Input: part model. Units: mm. Frame: model coordinates. Face numbers are marked on the shaded views. Coordinates: 2 decimals unless noted, no trailing zeros. Loops run counter-clockwise (first coordinate to the right, second up) from the corner with the lowest first, then second, coordinate; pieces in that order, holes last. Notation, with made-up numbers: (74, -14.75) -> (109, -14.75) arc R9 cw to (109, -7.75) -> close; hole circle Ø8 at (41, 74.5). An arc over 180 degrees is marked (long way). Answer as a JSON object with one key per item and string values.
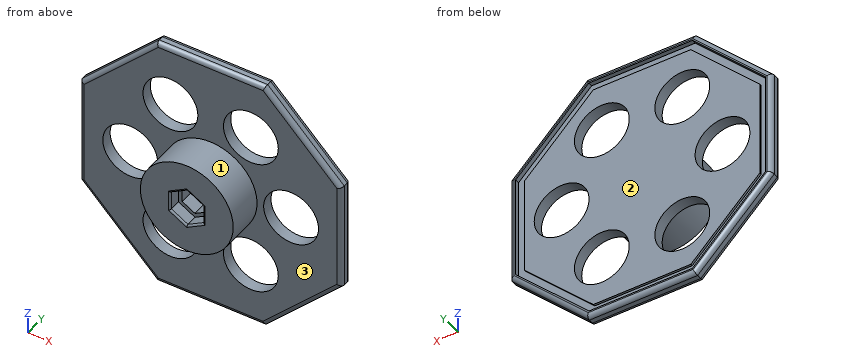
Autodesk Inventor part; units mm, degrees
ref_plane "YZ Plane" through (0, 0, 0) normal (1, 0, 0) x (0, 1, 0)
ref_plane "XZ Plane" through (0, 0, 0) normal (0, 1, 0) x (-1, 0, 0)
ref_plane "XY Plane" through (0, 0, 0) normal (0, 0, 1) x (1, 0, 0)
sketch "스케치3" plane through (0, 0, 0) normal (0, 1, 0) x (-1, 0, 0)
  line L0 (35.7919, -14.8255) -> (14.8255, -35.7919)
  line L1 (14.8255, -35.7919) -> (-14.8255, -35.7919)
  line L2 (-14.8255, -35.7919) -> (-35.7919, -14.8255)
  line L3 (-35.7919, -14.8255) -> (-35.7919, 14.8255)
  line L4 (-35.7919, 14.8255) -> (-14.8255, 35.7919)
  line L5 (-14.8255, 35.7919) -> (14.8255, 35.7919)
  line L6 (14.8255, 35.7919) -> (35.7919, 14.8255)
  line L7 (35.7919, 14.8255) -> (35.7919, -14.8255)
  line L8 (32.5919, -13.5) -> (13.5, -32.5919)
  line L9 (13.5, -32.5919) -> (-13.5, -32.5919)
  line L10 (-13.5, -32.5919) -> (-32.5919, -13.5)
  line L11 (-32.5919, -13.5) -> (-32.5919, 13.5)
  line L12 (-32.5919, 13.5) -> (-13.5, 32.5919)
  line L13 (-13.5, 32.5919) -> (13.5, 32.5919)
  line L14 (13.5, 32.5919) -> (32.5919, 13.5)
  line L15 (32.5919, 13.5) -> (32.5919, -13.5)
  point P0 (0, 0)
  point P1 (0, 0)
  point P2 (0, 0)
  point P3 (0, 0)
  dimension "d43" = 27
  dimension "d44" = 3.2
extrude "돌출2" add sketch "스케치3" along normal blind 3.7 contours L0 L1 L2 L3 L4 L5 L6 L7 | L8 L9 L10 L11 L12 L13 L14 L15
sketch "스케치4" plane through (0, 3.7, 0) normal (0, 1, 0) x (1, 0, 0)
  line L0 (13.5, -32.5919) -> (-13.5, -32.5919)
  line L1 (-13.5, -32.5919) -> (-32.5919, -13.5)
  line L2 (-32.5919, -13.5) -> (-32.5919, 13.5)
  line L3 (-32.5919, 13.5) -> (-13.5, 32.5919)
  line L4 (-13.5, 32.5919) -> (13.5, 32.5919)
  line L5 (13.5, 32.5919) -> (32.5919, 13.5)
  line L6 (32.5919, 13.5) -> (32.5919, -13.5)
  line L7 (32.5919, -13.5) -> (13.5, -32.5919)
  line L8 (-14.1627, 34.1919) -> (14.1627, 34.1919)
  line L9 (14.1627, 34.1919) -> (34.1919, 14.1627)
  line L10 (34.1919, 14.1627) -> (34.1919, -14.1627)
  line L11 (34.1919, -14.1627) -> (14.1627, -34.1919)
  line L12 (14.1627, -34.1919) -> (-14.1627, -34.1919)
  line L13 (-14.1627, -34.1919) -> (-34.1919, -14.1627)
  line L14 (-34.1919, -14.1627) -> (-34.1919, 14.1627)
  line L15 (-34.1919, 14.1627) -> (-14.1627, 34.1919)
  line L16 (-13.3343, 32.1919) -> (13.3343, 32.1919)
  line L17 (13.3343, 32.1919) -> (32.1919, 13.3343)
  line L18 (32.1919, 13.3343) -> (32.1919, -13.3343)
  line L19 (32.1919, -13.3343) -> (13.3343, -32.1919)
  line L20 (13.3343, -32.1919) -> (-13.3343, -32.1919)
  line L21 (-13.3343, -32.1919) -> (-32.1919, -13.3343)
  line L22 (-32.1919, -13.3343) -> (-32.1919, 13.3343)
  line L23 (-32.1919, 13.3343) -> (-13.3343, 32.1919)
  line L24 (-35.7919, 14.8255) -> (-35.7919, -14.8255)
  point P0 (0, 0)
  point P1 (0, 0)
  point P2 (0, 0)
  point P3 (0, 0)
  dimension "d7" = 27
  dimension "d60" = 1.6
  dimension "d61" = 2
extrude "돌출3" cut sketch "스케치4" against normal blind 1.2 contours L0 L1 L2 L3 L4 L5 L6 L7 | L8 L9 L10 L11 L12 L13 L14 L15 | L16 L17 L18 L19 L20 L21 L22 L23
sketch "스케치9" plane through (0, 2.5, 0) normal (0, 1, 0) x (1, 0, 0)
  line L0 (-13.3343, 32.1919) -> (13.3343, 32.1919)
  line L1 (13.3343, 32.1919) -> (32.1919, 13.3343)
  line L2 (32.1919, 13.3343) -> (32.1919, -13.3343)
  line L3 (32.1919, -13.3343) -> (13.3343, -32.1919)
  line L4 (13.3343, -32.1919) -> (-13.3343, -32.1919)
  line L5 (-13.3343, -32.1919) -> (-32.1919, -13.3343)
  line L6 (-32.1919, -13.3343) -> (-32.1919, 13.3343)
  line L7 (-32.1919, 13.3343) -> (-13.3343, 32.1919)
  line L8 (-14.1627, 34.1919) -> (14.1627, 34.1919)
  line L9 (-12.0917, 29.1919) -> (12.0917, 29.1919)
  line L10 (12.0917, 29.1919) -> (29.1919, 12.0917)
  line L11 (29.1919, 12.0917) -> (29.1919, -12.0917)
  line L12 (29.1919, -12.0917) -> (12.0917, -29.1919)
  line L13 (12.0917, -29.1919) -> (-12.0917, -29.1919)
  line L14 (-12.0917, -29.1919) -> (-29.1919, -12.0917)
  line L15 (-29.1919, -12.0917) -> (-29.1919, 12.0917)
  line L16 (-29.1919, 12.0917) -> (-12.0917, 29.1919)
  point P0 (0, 0)
  point P1 (0, 0)
  point P2 (0, 0)
  dimension "d46" = 2
  dimension "d47" = 3
extrude "돌출8" add sketch "스케치9" along normal blind 0.6 contours L0 L1 L2 L3 L4 L5 L6 L7 | L9 L10 L11 L12 L13 L14 L15 L16
fillet "모깎기1" radius 1.2 16 edges at (-35.7919, 3.7, 0) (-25.3087, 3.7, 25.3087) (0, 3.7, 35.7919) (25.3087, 3.7, 25.3087) (35.7919, 3.7, 0) (25.3087, 3.7, -25.3087) (0, 3.7, -35.7919) (-25.3087, 3.7, -25.3087) (25.3087, 0, 25.3087) (0, 0, 35.7919) (-25.3087, 0, 25.3087) (-35.7919, 0, 0) (-25.3087, 0, -25.3087) (0, 0, -35.7919) (25.3087, 0, -25.3087) (35.7919, 0, 0)
sketch "스케치11" plane through (0, 0, 0) normal (0, -1, 0) x (1, 0, 0)
  circle A0 centre (0, 0) radius 12.7
  dimension "d62" = 25.4
extrude "돌출11" add sketch "스케치11" along normal blind 10.16
sketch "스케치12" plane through (0, -10.16, 0) normal (0, -1, 0) x (1, 0, 0)
  circle A0 centre (0, 0) radius 4.5
  line L0 (4.5, 2.5981) -> (4.5, -2.5981)
  line L1 (4.5, -2.5981) -> (0, -5.1962)
  line L2 (0, -5.1962) -> (-4.5, -2.5981)
  line L3 (-4.5, -2.5981) -> (-4.5, 2.5981)
  line L4 (-4.5, 2.5981) -> (0, 5.1962)
  line L5 (0, 5.1962) -> (4.5, 2.5981)
  point P0 (2.25, 3.8971)
  point P1 (-2.25, 3.8971)
  point P2 (4.5, 0)
  point P3 (-4.5, 0)
  point P4 (-2.25, -3.8971)
  point P5 (2.25, -3.8971)
  dimension "d65" = 9
extrude "돌출12" cut sketch "스케치12" against normal blind 12
sketch "스케치13" plane through (0, 0, 0) normal (0, -1, 0) x (1, 0, 0)
  circle A0 centre (-22, 0) radius 7.5
  circle A1 centre (-11, -19.0526) radius 7.5
  circle A2 centre (11, -19.0526) radius 7.5
  circle A3 centre (22, 0) radius 7.5
  circle A4 centre (11, 19.0526) radius 7.5
  circle A5 centre (-11, 19.0526) radius 7.5
  point P0 (0, 0)
  dimension "d70" = 15
  dimension "d71" = 22
  dimension "d74" = 360
extrude "돌출13" cut sketch "스케치13" against normal up to surface (3.1 mm away)
sketch "스케치18" plane through (0, 1.84, 0) normal (0, -1, 0) x (1, 0, 0)
  line L0 (4.5, 2.5981) -> (4.5, -2.5981)
  line L1 (0, 5.1962) -> (4.5, 2.5981)
  line L2 (-4.5, 2.5981) -> (0, 5.1962)
  line L3 (-4.5, -2.5981) -> (-4.5, 2.5981)
  line L4 (0, -5.1962) -> (-4.5, -2.5981)
  line L5 (4.5, -2.5981) -> (0, -5.1962)
  line L6 (3.5, 2.0207) -> (3.5, -2.0207)
  line L7 (3.5, -2.0207) -> (0, -4.0415)
  line L8 (0, -4.0415) -> (-3.5, -2.0207)
  line L9 (-3.5, -2.0207) -> (-3.5, 2.0207)
  line L10 (-3.5, 2.0207) -> (0, 4.0415)
  line L11 (0, 4.0415) -> (3.5, 2.0207)
  point P0 (0, 0)
  point P1 (0, 0)
  dimension "d116" = 1
extrude "돌출14" add sketch "스케치18" along normal blind 8.5
fillet "모깎기2" radius 0.5 6 edges at (2.25, -10.16, 3.8971) (-2.25, -10.16, 3.8971) (4.5, -10.16, 0) (2.25, -10.16, -3.8971) (-2.25, -10.16, -3.8971) (-4.5, -10.16, 0)
equation "\"d85\" = 55deg"
equation "\"d105\" = 55deg"
properties part number "OV-PAM_top_2"
1. Section query B-B (x = -11). Return loops of the section in (y, z), plus the area to 3 significant figures.
Reply:
{"outline": "(-10.16, -6.35) -> (0, -6.35) -> (0, -11.55) -> (3.1, -11.55) -> (3.1, 11.55) -> (0, 11.55) -> (0, 6.35) -> (-10.16, 6.35) -> close; (0, -34.59) arc R1.2 ccw to (1.2, -35.79) -> (2.5, -35.79) arc R1.2 ccw to (3.7, -34.59) -> (3.7, -34.19) -> (2.5, -34.19) -> (2.5, -32.19) -> (3.1, -32.19) -> (3.1, -26.55) -> (0, -26.55) -> close; (0, 26.55) -> (3.1, 26.55) -> (3.1, 32.19) -> (2.5, 32.19) -> (2.5, 34.19) -> (3.7, 34.19) -> (3.7, 34.59) arc R1.2 ccw to (2.5, 35.79) -> (1.2, 35.79) arc R1.2 ccw to (0, 34.59) -> close", "area": "256 mm2"}
2. Section query C-C (z = 10). Return loops of the section in (x, y).
Reply:
{"outline": "(-35.79, 1.2) arc R1.2 ccw to (-34.59, 0) -> (-7.83, 0) -> (-7.83, -10.16) -> (7.83, -10.16) -> (7.83, 0) -> (34.59, 0) arc R1.2 ccw to (35.79, 1.2) -> (35.79, 2.5) arc R1.2 ccw to (34.59, 3.7) -> (34.19, 3.7) -> (34.19, 2.5) -> (32.19, 2.5) -> (32.19, 3.1) -> (-32.19, 3.1) -> (-32.19, 2.5) -> (-34.19, 2.5) -> (-34.19, 3.7) -> (-34.59, 3.7) arc R1.2 ccw to (-35.79, 2.5) -> close"}
3. Line query: line 1 along Z through (x, y) = (11, 1.25); line 2 along Z through (x, y) = (27.5, 1); line 3 along Y through (x, z) = (-22, -24.5). Output: solid intervals per line, ascending.
Reply:
{"line 1": "z = -35.79 to -26.55, -11.55 to 11.55, 26.55 to 35.79", "line 2": "z = -23.09 to -5.1, 5.1 to 23.09", "line 3": "y = 0 to 2.5"}
4. Pin query (flat end, axial travel): P1, Ø1, axis at y = 3, z = 5.5, coming from the -X side; P2, Ø5, axis at x = -24.5, z = -13, coming from the -Y side; P3, Ø17, axis at x = -11, z = -19.05, coming from the +Y side; P4, Ø0.9, axis at y = -8, z = 0, coming from the -X side. Return the tip coordinate at first contact, or that it passes through.
Reply:
{"P1": "stops at x = -35.79", "P2": "stops at y = 0", "P3": "stops at y = 3.1", "P4": "stops at x = -12.7"}
5. Mould query, pull axis X, two halves, no side actions, for the marked faces 1, 2 and 3. Classes: pulls with the +X half, pulls with the -X half, needs draft (parallel to the pull), parting line crosses it, or undercut.
Reply:
{"face 1": "parting line crosses it", "face 2": "undercut", "face 3": "needs draft"}
6. Section query D-D (x = 10.5). Return loops of the section in (y, z).
Reply:
{"outline": "(-10.16, -7.14) -> (0, -7.14) -> (0, -11.57) -> (3.1, -11.57) -> (3.1, 11.57) -> (0, 11.57) -> (0, 7.14) -> (-10.16, 7.14) -> close; (0, -34.59) arc R1.2 ccw to (1.2, -35.79) -> (2.5, -35.79) arc R1.2 ccw to (3.7, -34.59) -> (3.7, -34.19) -> (2.5, -34.19) -> (2.5, -32.19) -> (3.1, -32.19) -> (3.1, -26.54) -> (0, -26.54) -> close; (0, 26.54) -> (3.1, 26.54) -> (3.1, 32.19) -> (2.5, 32.19) -> (2.5, 34.19) -> (3.7, 34.19) -> (3.7, 34.59) arc R1.2 ccw to (2.5, 35.79) -> (1.2, 35.79) arc R1.2 ccw to (0, 34.59) -> close"}
7. Section query A-A (y = -3). Return loops of the section in (x, z), plus the area to 3 significant figures.
Reply:
{"outline": "circle Ø25.4 at (0, 0); hole (-3.5, -2.02) -> (0, -4.04) -> (3.5, -2.02) -> (3.5, 2.02) -> (0, 4.04) -> (-3.5, 2.02) -> close", "area": "464 mm2"}
